```python
from build123d import *

# Parameters (mm, degrees)
EXTRUDE_1_DEPTH     = 162.2
SKETCH_4_R          = 3
EXTRUDE_2_DEPTH     = 5
SKETCH_5_R          = 3
EXTRUDE_3_DEPTH     = 5
SKETCH_6_W          = 1
SKETCH_6_H          = 0.5
EXTRUDE_4_DEPTH     = 162.2
SKETCH_3_R          = 3
SKETCH_3_R_2        = 7
SKETCH_3_R_3        = 4
CUT_EXTRUDE_1_DEPTH = 40


with BuildPart() as part:
    # 스케치1 → 보스-돌출1 (new body)
    with BuildSketch(Plane.XY):
        Polygon((0, -20), (25, -20), (25, -17), (3, -17), (3, 17), (25, 17), (25, 20), (0, 20), align=None)
    extrude(amount=EXTRUDE_1_DEPTH)

    # 스케치4 → 보스-돌출2 (add)
    with BuildSketch(Plane.XY.offset(162.2)):
        with BuildLine():
            Line((0, 33), (0, 20))
            Line((0, 20), (15, 20))
            Line((15, 20), (15, 33))
            ThreePointArc((15, 33), (7.5, 40.5), (0, 33))
        make_face()
        with Locations((7.5, 33)):
            Circle(SKETCH_4_R, mode=Mode.SUBTRACT)
    extrude(amount=-EXTRUDE_2_DEPTH)

    # 스케치5 → 보스-돌출3 (add)
    with BuildSketch(Plane(origin=(0, 0, 0), x_dir=(-1, 0, 0), z_dir=(0, 0, -1))):
        with BuildLine():
            ThreePointArc((0, 33), (-7.5, 40.5), (-15, 33))
            Line((-15, 33), (-15, 20))
            Line((-15, 20), (0, 20))
            Line((0, 20), (0, 33))
        make_face()
        with Locations((-7.5, 33)):
            Circle(SKETCH_5_R, mode=Mode.SUBTRACT)
    extrude(amount=-EXTRUDE_3_DEPTH)

    # 스케치6 → 보스-돌출4 (add)
    with BuildSketch(Plane.XY.offset(162.2)):
        with Locations((24.5, -16.75)):
            Rectangle(SKETCH_6_W, SKETCH_6_H)
    extrude(amount=-EXTRUDE_4_DEPTH)

    # 스케치3 → 컷-돌출1 (cut)
    with BuildSketch(Plane(origin=(0, 20, 0), x_dir=(1, 0, 0), z_dir=(0, 1, 0))):
        with Locations((14, -142.2)):
            Circle(SKETCH_3_R)
        with Locations((14, -128.7)):
            Circle(SKETCH_3_R)
        with Locations((14, -115.2)):
            Circle(SKETCH_3_R)
        with Locations((14, -101.7)):
            Circle(SKETCH_3_R)
        with Locations((14, -74.7)):
            Circle(SKETCH_3_R)
        with Locations((14, -88.2)):
            Circle(SKETCH_3_R)
        with Locations((14, -45)):
            Circle(SKETCH_3_R_2)
        with Locations((14, -25)):
            Circle(SKETCH_3_R_2)
        with Locations((14, -61.2)):
            Circle(SKETCH_3_R_3)
    extrude(amount=-CUT_EXTRUDE_1_DEPTH, mode=Mode.SUBTRACT)


solid = part.part
```
Could you check a few things on this model? Use its own coordinates, in mm. A direction names the side the tool comes from. Round coordinates to 2 decimals unless told otherwise and drop trailing zeros. Loops run counter-clockwise (first coordinate to the right, second up) from the corner with the lowest first, then second, coordinate; pieces in that order, holes last.
Q1. On a 3-axis mill with a long thin cutter (end or side, diameter ignored), from which of +Z, -Z, +X, -X, +Y, -Y can I reach the whole of each face in a straight line? I mean faces 1 (the flat face through (15, 27, 2)), 2 (the cylindrical face through (11.6, 18.5, 90)), 3 (the flat face through (7, 28, 157.2)). Say none if no direction works.
Q2. I want a section at A-A (z = 45). Write out the boundary of the cut face in (x, y).
Q3. I want a section at C-C (y = 12). Write out the boundary of the cut face in (x, z).
Q4. I want a section at B-B (z = 74.7). Write out the boundary of the cut face in (x, y).
Q5. Please list where these lines run through material, in increasing order: L1, parallel to Y at x = 3.75, z = 125.5; L2, parallel to X at y = 18.65, z = 88.2; L3, parallel to X at y = 18.3, z = 25.
Q6. For P1, Ø4, axis at x = 15.5, z = 78.5, coming from the +Y side; P2, Ø5, axis at x = 14, z = 142.2, coming from the -Y side, each with a flat end and sliding along its axis, tell me the tip position at first contact or that it passes through.
Q7. Thinking about a two-plate mould opening in Y: for faces 4 (the cylindrical face through (7.34, 40.5, 2.46)), 5 (the flat face through (14, 17, 80)), 6 (the cylindrical face through (13.609, -18.479, 139.226)), which applies, pulls with the +Y half, pulls with the -Y half, needs draft (parallel to the pull), parting line crosses it, or undercut?
Answer below:
1. face 1: +Z, -Z, +X, +Y
1. face 2: +Y, -Y
1. face 3: +X, -X, +Y
2. outline: (0, -20) - (7, -20) - (7, -17) - (3, -17) - (3, 17) - (7, 17) - (7, 20) - (0, 20) - close; (21, -20) - (25, -20) - (25, -16.5) - (24, -16.5) - (24, -17) - (21, -17) - close; (21, 17) - (25, 17) - (25, 20) - (21, 20) - close
3. outline: (0, 0) - (3, 0) - (3, 162.2) - (0, 162.2) - close
4. outline: (0, -20) - (11, -20) - (11, -17) - (3, -17) - (3, 17) - (11, 17) - (11, 20) - (0, 20) - close; (17, -20) - (25, -20) - (25, -16.5) - (24, -16.5) - (24, -17) - (17, -17) - close; (17, 17) - (25, 17) - (25, 20) - (17, 20) - close
5. L1: y = -20 to -17, 17 to 20
5. L2: x = 0 to 11, 17 to 25
5. L3: x = 0 to 7, 21 to 25
6. P1: stops at y = 20
6. P2: passes through
7. face 4: pulls with the +Y half
7. face 5: undercut
7. face 6: needs draft
